Design review of the part shown in the three views and the two pictorial views. Dimensions are in mm from the part's minimum x, y and z. Coordinates: 2 decimals unless noted, no trailing zeros. Loops run counter-clockwise (first coordinate to the right, second up) from the corner with the lowest first, then second, coordinate; pieces in that order, holes last. Notation, with made-up numbers: (-36.75, 32.5) - (22.25, 32.5) arc R21 cw to (22.25, 44.5) - close; hole circle Ø11 at (1, 61). An arc over 180 degrees is marked (long way). One line per item, written item: value. Start each with the question number.
1. To check wall thickness, follow line 1 (Z direction, x = 13.5, y = 15.5); line 2 (X direction, y = 99, z = 64.5); line 3 (Z direction, x = 13.75, y = 26) (1 decimal). State the ranges of each line that lie inside material, in increasing order. Write a range as from..to.
2. Take a section at C-C, the plane y = 30. State the section outline as (x, z) points.
3. Insertion check: pin 1 (2.5 mm diameter, centred on x = 11.5, z = 66.5, fed in from +Y); pin 2 (4 mm diameter, centred on y = 68, z = 69.5, fed in from +X); pin 3 (8.5 mm diameter, centred on y = 79.5, z = 69, fed in from -X). Each pin has a flat end and moves straight along its axis. Give the tip position at first contact, or say it passes through.
4. Take a section at A-A, the plane x = 7.75. State the section outline as (y, z) points (1 decimal), and give its area (3 significant figures).
5. Take a section at B-B, the plane y = 46. State the section outline as (x, z) points, and give its area (3 significant figures).
6. Take a section at D-D, the plane x = 21. State the section outline as (y, z) points.
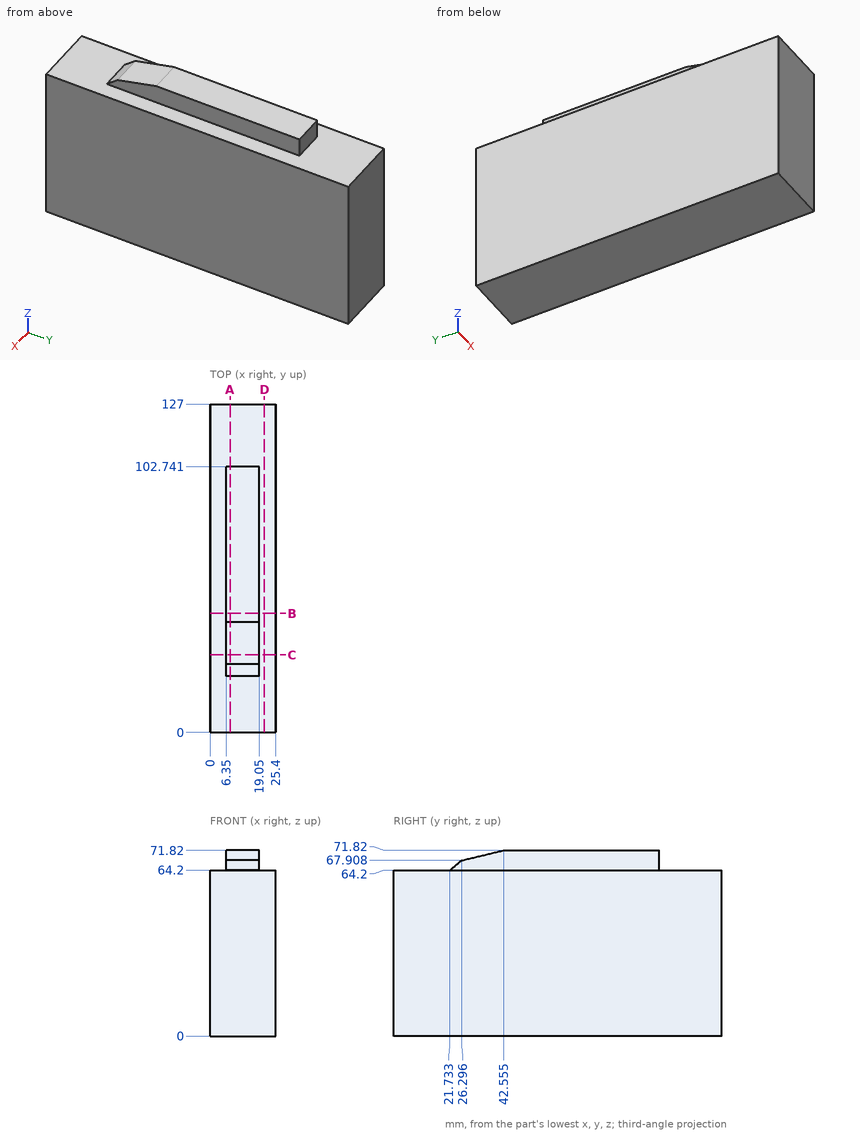
Solutions:
1. line 1: 0..64.2
1. line 2: 6.35..19.05
1. line 3: 0..67.7
2. outline: (0, 0) - (25.4, 0) - (25.4, 64.2) - (19.05, 64.2) - (19.05, 68.8) - (6.35, 68.8) - (6.35, 64.2) - (0, 64.2) - close
3. pin 1: y = 102.74
3. pin 2: x = 19.05
3. pin 3: x = 6.35
4. outline: (0, 0) - (127, 0) - (127, 64.2) - (102.7, 64.2) - (102.7, 71.8) - (42.6, 71.8) - (26.3, 67.9) - (21.7, 64.2) - (0, 64.2) - close
4. area: 8,710 mm2
5. outline: (0, 0) - (25.4, 0) - (25.4, 64.2) - (19.05, 64.2) - (19.05, 71.82) - (6.35, 71.82) - (6.35, 64.2) - (0, 64.2) - close
5. area: 1,730 mm2
6. outline: (0, 0) - (127, 0) - (127, 64.2) - (0, 64.2) - close
